Check sheet for the drawn part. Datum: minimum x, y, z corner. Units: mm. Coordinates: 2 decimals unless noted, no trailing zeros. Write each loop counter-clockwise with the first axis right and the second up, starting at its lowest first coordinate (ties: lowest second). Pieces come first, ordered by that corner, then holes. Notation, with made-up numbers: (-16, -6) -> (-12, -6) arc R19 ccw to (-12, -2) -> close; hole circle Ø7 at (-17, 33). An arc over 180 degrees is marked (long way). Write each question's results on one line, items separated by ' | '. Start each with the question number.
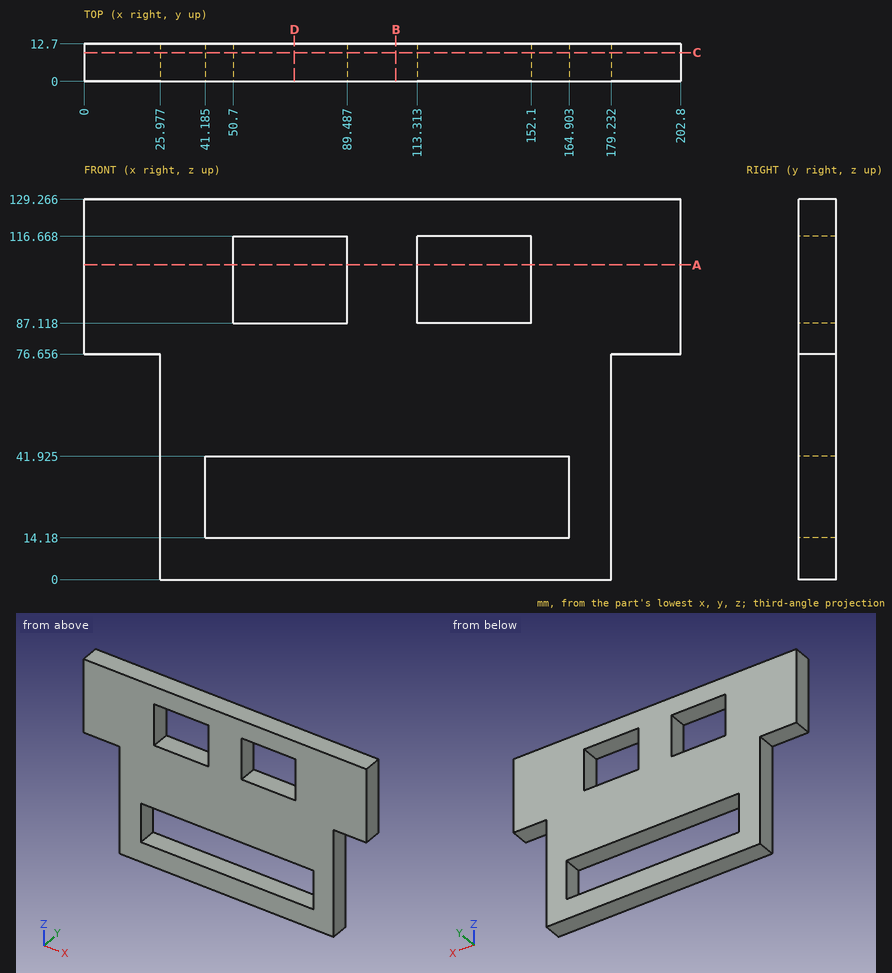
1. Sectioned sample at A-A on z = 107. Record the cut outline in (x, y), plus the area to 3 significant figures.
2. Depth check by flat-ended pin: pin 1 Ø6.5 at (y, z) = (5.5, 25.5) entering from +X; pin 2 Ø6.5 at (x, y) = (12, 8.5) entering from -Z. Enter the tip coordinate at first touch or a pass-through.
3. Sectioned sample at D-D on x = 71.5. Record the cut outline in (y, z) (1 decimal).
4. Sectioned sample at B-B on x = 106. Record the cut outline in (y, z) (1 decimal), plus the area to 3 significant figures.
5. Sectioned sample at C-C on y = 9.75. Record the cut outline in (x, z) (1 decimal), plus the area to 3 significant figures.
6. Material ranges on probe 1 along Z at (x, y) = (129, 11.25) (1 decimal); probe 2 along X at (y, z) = (1.75, 93); probe 3 along Z at (x, y) = (156, 4.5) (1 decimal), recorded low to high. Write a range as from..to.
Computed values:
1) outline: (0, 0) -> (50.7, 0) -> (50.7, 12.7) -> (0, 12.7) -> close; (89.49, 0) -> (113.31, 0) -> (113.31, 12.7) -> (89.49, 12.7) -> close; (152.1, 0) -> (202.8, 0) -> (202.8, 12.7) -> (152.1, 12.7) -> close | area: 1,590 mm^2
2) pin 1: stops at x = 179.23 | pin 2: stops at z = 76.66
3) outline: (0, 0) -> (12.7, 0) -> (12.7, 14.2) -> (0, 14.2) -> close; (0, 41.9) -> (12.7, 41.9) -> (12.7, 87.1) -> (0, 87.1) -> close; (0, 116.7) -> (12.7, 116.7) -> (12.7, 129.3) -> (0, 129.3) -> close
4) outline: (0, 0) -> (12.7, 0) -> (12.7, 14.2) -> (0, 14.2) -> close; (0, 41.9) -> (12.7, 41.9) -> (12.7, 129.3) -> (0, 129.3) -> close | area: 1,290 mm^2
5) outline: (0, 76.7) -> (26, 76.7) -> (26, 0) -> (179.2, 0) -> (179.2, 76.7) -> (202.8, 76.7) -> (202.8, 129.3) -> (0, 129.3) -> close; hole (41.2, 14.2) -> (164.9, 14.2) -> (164.9, 41.9) -> (41.2, 41.9) -> close; hole (50.7, 87.1) -> (89.5, 87.1) -> (89.5, 116.7) -> (50.7, 116.7) -> close; hole (113.3, 87.1) -> (152.1, 87.1) -> (152.1, 116.7) -> (113.3, 116.7) -> close | area: 16,700 mm^2
6) probe 1: z = 0..14.2, 41.9..87.1, 116.7..129.3 | probe 2: x = 0..50.7, 89.49..113.31, 152.1..202.8 | probe 3: z = 0..14.2, 41.9..129.3
